from build123d import *

# Parameters (mm, degrees)
BASE_EXTRUDE_DEPTH = 3


with BuildPart() as part:
    # Sketch1 → Base-Extrude (new body)
    with BuildSketch(Plane.XY):
        with BuildLine():
            Line((254.458999609, 72.42410604), (254.458999609, 68.312175266))
            Line((254.458999609, 68.312175266), (249.057113985, 71.99161005))
            Line((249.057113985, 71.99161005), (247.368253343, 69.512144436))
            Line((247.368253343, 69.512144436), (263.523901664, 58.507902857))
            ThreePointArc((263.523901664, 58.507902857), (271.838397848, 49.089575752), (278.059793662, 38.174908264))
            ThreePointArc((278.059793662, 38.174908264), (277.460971595, 35.494168544), (275.801504518, 33.305305293))
            ThreePointArc((275.801504518, 33.305305293), (272.168235705, 35.752461976), (267.87122217, 36.603868337))
            Line((267.87122217, 36.603868337), (266.553980851, 33.3090367))
            Line((266.553980851, 33.3090367), (251.02719612, 41.33883075))
            Line((251.02719612, 41.33883075), (245.072593427, 26.565797378))
            Line((245.072593427, 26.565797378), (230.827204858, 32.233531984))
            Line((230.827204858, 32.233531984), (225.897587097, 35.291364614))
            ThreePointArc((225.897587097, 35.291364614), (223.417826754, 38.317877983), (223.856638727, 42.205864427))
            Line((223.856638727, 42.205864427), (233.34569838, 36.950163447))
            Line((233.34569838, 36.950163447), (234.799244804, 39.574511517))
            Line((234.799244804, 39.574511517), (223.290021138, 45.949119784))
            ThreePointArc((223.290021138, 45.949119784), (223.201365162, 51.301598344), (224.516481401, 56.490755877))
            ThreePointArc((224.516481401, 56.490755877), (226.27528444, 67.636113231), (235.821369896, 73.651479483))
            Line((235.821369896, 73.651479483), (240.358475054, 70.837802847))
            Line((240.358475054, 70.837802847), (245.989993101, 76.519880328))
            ThreePointArc((245.989993101, 76.519880328), (250.765877804, 75.591430608), (254.458999609, 72.42410604))
        make_face()
        Polygon((240.093331419, 55.591825093), (257.438617194, 45.634864644), (255.945073126, 43.033071777), (238.599787351, 52.990032226), align=None, mode=Mode.SUBTRACT)
    extrude(amount=BASE_EXTRUDE_DEPTH)


solid = part.part
Work out the finished part from the listing and answer in its coordinate system (mm). A direction names the side the tool comes from. Coordinates: 2 decimals unless noted, no trailing zeros. Write each loop counter-clockwise with the first axis right and the second up, starting at its lowest first coordinate (ties: lowest second). Pieces come first, ordered by that corner, then holes. Notation, with made-up numbers: M 22.25,33.5 L 80.25,33.5 A20 ccw 80.25,69.5 Z; hole C -33,41 d4. An arc over 180 degrees is marked long. Use one line per item in the form item = value. Start each with the question number.
1. The part is cut by section B-B (x = 253). Give the vertices of the cut face in (y, z), plus the area to 3 significant figures.
2. The part is cut by section D-D (x = 244). Give the vertices of the cut face in (y, z).
3. The part is cut by section C-C (y = 36). Give the vertices of the cut face in (x, z), plus the area to 3 significant figures.
4. Straight lines are drawn through the part: probe 1 along Y at (x, z) = (246.5, 2.65); probe 2 along X at (y, z) = (71.5, 1.95); probe 3 along Y at (x, z) = (239, 2.15). For each, find the intervals that lie inside material, in ascending order. Write a range as from..to.
5. The part is cut by section A-A (z = 2.3). Give the vertices of the cut face in (x, y), plus the area to 3 significant figures.
6. Each of these flat-tipped pins is pushed along its axis until it touches: P1, Ø1, axis at x = 231.5, z = 2.5, coming from the +Y side; P2, Ø1, axis at x = 253, z = 1, coming from the -Y side; P3, Ø1.5, axis at x = 238.5, z = 2, coming from the -Y side. Where does it stop, or does it pass through?
7. A tool of negligible diameter and unlimited length cuts with its end or side. For faces 1 (the face through (223.193, 51.227, 1.479)), 2 (the face through (229.125, 42.717, 1.479)), 3 (the face through (238.058, 72.264, 1.479)), 4 (the face through (272.225, 35.729, 1.479)), from which of +Z, -Z, +X, -X, +Y, -Y can it reach the whole face along a straight path? Write none if from no direction.
8. The mould has two halves that part along X. Classify faces 5 (the face through (277.477, 35.529, 1.479)), 6 (the face through (245, 46, 3)), 7 (the face through (248.092, 34.056, 1.479)), 8 (the face through (223.434, 38.264, 1.479)): released by +X, released by -X, zero draft, split by the parting line, or undercut.
Evaluation:
q1.outline = M 40.32,0 L 44.72,0 L 44.72,3 L 40.32,3 Z; M 48.18,0 L 65.68,0 L 65.68,3 L 48.18,3 Z; M 69.31,0 L 74.09,0 L 74.09,3 L 69.31,3 Z
q1.area = 80.0 mm^2
q2.outline = M 26.99,0 L 49.89,0 L 49.89,3 L 26.99,3 Z; M 53.35,0 L 74.51,0 L 74.51,3 L 53.35,3 Z
q3.outline = M 224.88,0 L 248.88,0 L 248.88,3 L 224.88,3 Z; M 261.35,0 L 267.63,0 L 267.63,3 L 261.35,3 Z; M 271.52,0 L 277.67,0 L 277.67,3 L 271.52,3 Z
q3.area = 109 mm^2
q4.probe_1 = 30.11..48.45, 51.91..76.54
q4.probe_2 = 230.13..239.29, 241.01..248.72, 249.78..254.46
q4.probe_3 = 28.98..52.76, 53.69..71.68
q5.outline = M 223.29,45.95 L 234.8,39.57 L 233.35,36.95 L 223.86,42.21 A5.03 ccw 225.9,35.29 L 230.83,32.23 L 245.07,26.57 L 251.03,41.34 L 266.55,33.31 L 267.87,36.6 A11.1 cw 275.8,33.31 A6.45 ccw 278.06,38.17 A61.34 ccw 263.52,58.51 L 247.37,69.51 L 249.06,71.99 L 254.46,68.31 L 254.46,72.42 A9.52 ccw 245.99,76.52 L 240.36,70.84 L 235.82,73.65 A13.65 ccw 224.52,56.49 A20.28 ccw Z; hole M 238.6,52.99 L 255.95,43.03 L 257.44,45.63 L 240.09,55.59 Z
q5.area = 1,540 mm^2
q6.P1 = 72.54
q6.P2 = 40.06
q6.P3 = 28.88
q7.face_1 = +Z, -Z, -X
q7.face_2 = +Z, -Z
q7.face_3 = +Z, -Z, +Y
q7.face_4 = +Z, -Z, -Y
q8.face_5 = released by +X
q8.face_6 = zero draft
q8.face_7 = undercut
q8.face_8 = released by -X
